```python
from build123d import *

# Parameters (mm, degrees)
SKETCH1_W               = 104.449895642
SKETCH1_H               = 44.57694291
BOSS_EXTRUDE1_DEPTH     = 3
SKETCH3_R               = 3.1
CUT_EXTRUDE1_DEPTH      = 10
SKETCH4_R               = 1.5
CUT_EXTRUDE2_DEPTH      = 10
MIRROR2_COPY_1_SKETCH_R = 1.5
MIRROR2_COPY_1_DEPTH    = 10
CUT_EXTRUDE3_DEPTH      = 57.861420442
CUT_EXTRUDE4_DEPTH      = 57.861420442
CUT_EXTRUDE5_DEPTH      = 57.861420442


with BuildPart() as part:
    # Sketch1 → Boss-Extrude1 (new body)
    with BuildSketch(Plane.XY):
        Rectangle(SKETCH1_W, SKETCH1_H)
    extrude(amount=BOSS_EXTRUDE1_DEPTH)

    # Sketch3 → Cut-Extrude1 (cut)
    with BuildSketch(Plane.XY.offset(3)):
        with Locations((19.775052179, 0)):
            Circle(SKETCH3_R)
        with Locations((-17.724947821, 0)):
            Circle(SKETCH3_R)
        with Locations((-40.224947821, 0)):
            Circle(SKETCH3_R)
    extrude(amount=-CUT_EXTRUDE1_DEPTH, mode=Mode.SUBTRACT)

    # Sketch4 → Cut-Extrude2 (cut)
    with BuildSketch(Plane.XY.offset(3)):
        with Locations((-48.447057672, 18.248177723)):
            Circle(SKETCH4_R)
    cut_extrude2 = extrude(amount=-CUT_EXTRUDE2_DEPTH, mode=Mode.SUBTRACT)

    # Mirror1: Cut-Extrude2 across plane
    add(cut_extrude2.mirror(Plane(origin=(0, 0, 0), x_dir=(0, 0, 1), z_dir=(1, 0, 0))), mode=Mode.SUBTRACT)

    # Mirror2: Cut-Extrude2 across plane
    add(cut_extrude2.mirror(Plane.ZX), mode=Mode.SUBTRACT)

    # Mirror2 copy 1 sketch → Mirror2 copy 1 (cut)
    with BuildSketch(Plane(origin=(0, 0, 3), x_dir=(-1, 0, 0), z_dir=(0, 0, 1))):
        with Locations((-48.447057672, 18.248177723)):
            Circle(MIRROR2_COPY_1_SKETCH_R)
    extrude(amount=-MIRROR2_COPY_1_DEPTH, mode=Mode.SUBTRACT)

    # Sketch5 → Cut-Extrude3 (cut, through all)
    with BuildSketch(Plane.XY.offset(3)):
        with BuildLine():
            Line((-41.337055779, 17.064455462), (-20.413840907, 17.064455462))
            Line((-20.413840907, 17.064455462), (-20.413840907, 6.345404524))
            ThreePointArc((-20.413840907, 6.345404524), (-22.338128988, 5.11985001), (-23.756861687, 3.333214622))
            Line((-23.756861687, 3.333214622), (-34.356294023, 3.333214622))
            ThreePointArc((-34.356294023, 3.333214622), (-39.005765332, 6.638148173), (-44.52617342, 5.201045612))
            Line((-44.52617342, 5.201045612), (-44.52617342, 12.200038175))
            ThreePointArc((-44.52617342, 12.200038175), (-42.419143342, 14.296270065), (-41.337055779, 17.064455462))
        make_face()
    cut_extrude3 = extrude(amount=-CUT_EXTRUDE3_DEPTH, mode=Mode.SUBTRACT)

    # Mirror3: Cut-Extrude3 across plane
    add(cut_extrude3.mirror(Plane.ZX), mode=Mode.SUBTRACT)

    # Sketch6 → Cut-Extrude4 (cut, through all)
    with BuildSketch(Plane.XY.offset(3)):
        with BuildLine():
            Line((-13.015804561, -17.064455462), (-13.015804561, -6.345404524))
            ThreePointArc((-13.015804561, -6.345404524), (-11.600072812, -4.992604025), (-10.56046116, -3.333214622))
            Line((-10.56046116, -3.333214622), (14.157752022, -3.333214622))
            ThreePointArc((14.157752022, -3.333214622), (15.888120713, -5.249394684), (18.225787128, -6.345404524))
            Line((18.225787128, -6.345404524), (18.225787128, -17.064455462))
            Line((18.225787128, -17.064455462), (-13.015804561, -17.064455462))
        make_face()
    cut_extrude4 = extrude(amount=-CUT_EXTRUDE4_DEPTH, mode=Mode.SUBTRACT)

    # Mirror4: Cut-Extrude4 across plane
    add(cut_extrude4.mirror(Plane.ZX), mode=Mode.SUBTRACT)

    # Sketch7 → Cut-Extrude5 (cut, through all)
    with BuildSketch(Plane.XY.offset(3)):
        with BuildLine():
            Line((20.845739993, -6.345404524), (20.845739993, -17.064455462))
            Line((20.845739993, -17.064455462), (42.074566495, -17.064455462))
            ThreePointArc((42.074566495, -17.064455462), (44.778043986, -12.905127961), (49.630779933, -11.875686546))
            Line((49.630779933, -11.875686546), (49.630779933, -3.333214622))
            Line((49.630779933, -3.333214622), (25.279614946, -3.333214622))
            ThreePointArc((25.279614946, -3.333214622), (23.391238299, -5.322943633), (20.845739993, -6.345404524))
        make_face()
    cut_extrude5 = extrude(amount=-CUT_EXTRUDE5_DEPTH, mode=Mode.SUBTRACT)

    # Mirror5: Cut-Extrude5 across plane
    add(cut_extrude5.mirror(Plane.ZX), mode=Mode.SUBTRACT)


solid = part.part
```
Work out the finished part from the listing and answer in its coordinate system (mm). A direction names the side the tool comes from. Give positions to 0.01 mm unless a question says otherwise; leave off trailing zeros. Write each loop counter-clockwise with the first axis right and the second up, starting at its lowest first coordinate (ties: lowest second). Pieces come first, ordered by that corner, then holes. Notation, with made-up numbers: (-38.75, -12) - (-12.75, -12) arc R21 ccw to (-12.75, 18) - close; hole circle Ø8 at (-1.75, 26). An arc over 180 degrees is marked (long way). Use one line per item in the form item = value.
1. Determine the mould class of faces 3 (the face through (-1, -22.288, 1)), 4 (the face through (-1, 0, 0)), 5 (the face through (38, 3.333, 2)) for opening direction Y: released by +Y, released by -Y, zero draft, split by the parting line, or undercut.
Filled in:
face_3 = released by -Y
face_4 = zero draft
face_5 = undercut
2. A cutting plane is placed at A-A (y = 0). Write down the section's boundary in (x, z), and give its area (3 significant figures).
Filled in:
outline = (-52.22, 0) - (-43.32, 0) - (-43.32, 3) - (-52.22, 3) - close; (-37.12, 0) - (-20.82, 0) - (-20.82, 3) - (-37.12, 3) - close; (-14.62, 0) - (16.68, 0) - (16.68, 3) - (-14.62, 3) - close; (22.88, 0) - (52.22, 0) - (52.22, 3) - (22.88, 3) - close
area = 258 mm^2
3. This flat-tipped pin is pushed along its axis until it touches: pin 1 Ø5 at (x, y) = (19.78, 0) entering from +Z. Where does it stop, or does it pass through?
Filled in:
pin_1 = through
4. A cutting plane is placed at D-D (x = -22.5). Write down the section's boundary in (y, z), and give its area (3 significant figures).
Filled in:
outline = (-22.29, 0) - (-17.06, 0) - (-17.06, 3) - (-22.29, 3) - close; (-4.97, 0) - (4.97, 0) - (4.97, 3) - (-4.97, 3) - close; (17.06, 0) - (22.29, 0) - (22.29, 3) - (17.06, 3) - close
area = 61.2 mm^2
5. For faces 1 (the face through (20.846, 12, 2)), 2 (the face through (-1, 22.288, 1)), determine the directions among +Z, -Z, +X, -X, +Y, -Y from which every point of the face is accessible in a straight line to the end or side of a thin tool.
Filled in:
face_1 = +Z, -Z
face_2 = +Z, -Z, +X, -X, +Y
6. A cutting plane is placed at B-B (x = 0.5). Write down the section's boundary in (y, z).
Filled in:
outline = (-22.29, 0) - (-17.06, 0) - (-17.06, 3) - (-22.29, 3) - close; (-3.33, 0) - (3.33, 0) - (3.33, 3) - (-3.33, 3) - close; (17.06, 0) - (22.29, 0) - (22.29, 3) - (17.06, 3) - close
7. Consider L1, parallel to Y at x = 7.5, z = 1.2; L2, parallel to X at y = 10.5, z = 1; L3, parallel to Y at x = 21, z = 0.65. Determine where each line is inside the solid, lowest interval first.
Filled in:
L1 = -22.29 to -17.06, -3.33 to 3.33, 17.06 to 22.29
L2 = -52.22 to -44.53, -20.41 to -13.02, 18.23 to 20.85, 49.63 to 52.22
L3 = -22.29 to -17.06, -6.32 to -2.85, 2.85 to 6.32, 17.06 to 22.29
8. A cutting plane is placed at C-C (y = -8). Write down the section's boundary in (x, z), and give its area (3 significant figures).
Filled in:
outline = (-52.22, 0) - (-44.53, 0) - (-44.53, 3) - (-52.22, 3) - close; (-20.41, 0) - (-13.02, 0) - (-13.02, 3) - (-20.41, 3) - close; (18.23, 0) - (20.85, 0) - (20.85, 3) - (18.23, 3) - close; (49.63, 0) - (52.22, 0) - (52.22, 3) - (49.63, 3) - close
area = 60.9 mm^2
